Autodesk Inventor part; units mm, degrees
sketch "Sketch1" plane through (0, 0, 0) normal (0, 0, 1) x (1, 0, 0)
  circle A0 centre (0, 0) radius 6
  dimension "d0" = 12
extrude "Extrusion1" add sketch "Sketch1" along normal mid plane 128
sketch "Sketch2" plane through (0, 0, -64) normal (0, 0, -1) x (-1, 0, 0)
  line L0 (0, 10) -> (8.6603, 5)
  line L1 (8.6603, 5) -> (8.6603, -5)
  line L2 (8.6603, -5) -> (0, -10)
  line L3 (0, -10) -> (-8.6603, -5)
  line L4 (-8.6603, -5) -> (-8.6603, 5)
  line L5 (-8.6603, 5) -> (0, 10)
  point P0 (0, 0)
  point P1 (0, 0)
  dimension "d3" = 10
extrude "Extrusion2" add sketch "Sketch2" along normal blind 5
thread "Thread1"
chamfer "Chamfer1" distance 2 angle 45 1 edges at (-6, 0, 64)
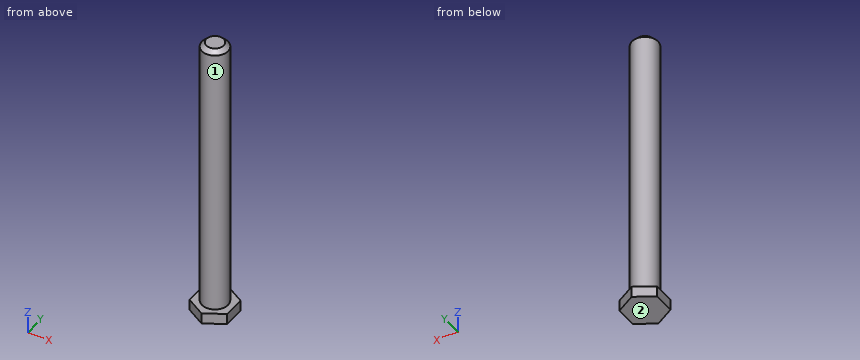
CAD build for the part. Positions are in the model's coordinates, mm. Face numbers are marked on the shaded views. A direction names the side the tool comes from. Round coordinates to 2 decimals unless told otherwise and drop trailing zeros. Write each loop counter-clockwise with the first axis right and the second up, starting at its lowest first coordinate (ties: lowest second). Pieces come first, ordered by that corner, then holes. Notation, with made-up numbers: M 2,80.5 L 47,80.5 A22 ccw 47,117.5 Z; hole C -2,13.25 d6. An arc over 180 degrees is marked long. Use a Markdown table: item, result. Add a question column.
1. Drill centre lines: probe 1 along Z at (x, y) = (6, 1.5); probe 2 along X at (y, z) = (0.25, -50.5). Where is each one in solid material? Low to high.
2. Slice it at A-A on y = 0. Give the cut face in (x, z), then the cut area to 3 significant figures.
3. Flat gauge pins, fed straight in: P1, Ø6, axis at y = -3.5, z = 11.5, coming from the +X side; P2, Ø10, axis at x = -1, z = -52.5, coming from the +Y side; P3, Ø8, axis at x = 5, z = 5, coming from the -Y side. Where does each tip first touch, or does it go through?
4. 3-axis set-ups, long thin cutter, end or side, ignore diameter. For the marked faces 1 and 2: which of +Z, -Z, +X, -X, +Y, -Y reach the whole face in a straight line?
5. Slice it at B-B on z = -34. Give the cut face in (x, y), then the cut area to 3 significant figures.
Reply:
| question | item | result |
|---|---|---|
| 1 | probe 1 | z = -69 to -64 |
| 1 | probe 2 | x = -5.99 to 5.99 |
| 2 | outline | M -8.66,-69 L 8.66,-69 L 8.66,-64 L 6,-64 L 6,62 L 4,64 L -4,64 L -6,62 L -6,-64 L -8.66,-64 Z |
| 2 | area | 1,620 mm^2 |
| 3 | P1 | stops at x = 5.98 |
| 3 | P2 | stops at y = 6 |
| 3 | P3 | stops at y = -5.92 |
| 4 | face 1 | +Z |
| 4 | face 2 | -Z, +X, -X, +Y, -Y |
| 5 | outline | C 0,0 d12 |
| 5 | area | 113 mm^2 |
